```python
from build123d import *

# Parameters (mm, degrees)
F0_W     = 76.2
F0_H     = 25.4
F1_DEPTH = 12.7
F2_W     = 12.7
F2_H     = 12.7
F3_DEPTH = 63.5
F4_R     = 3.175
F5_DEPTH = 50.8


with BuildPart() as f1:
    # F0 (on Top) → F1 (new body)
    with BuildSketch(Plane.XY):
        Rectangle(F0_W, F0_H)
    extrude(amount=F1_DEPTH)

    # F2 (on face) → F3 (join)
    with BuildSketch(Plane.XY.offset(12.7)):
        Rectangle(F2_W, F2_H)
    extrude(amount=F3_DEPTH)

    # F4 (on face) → F5 (join)
    with BuildSketch(Plane.XZ.offset(6.35)):
        with Locations((0, 63.5)):
            Circle(F4_R)
    extrude(amount=F5_DEPTH)


solid = f1.part
```
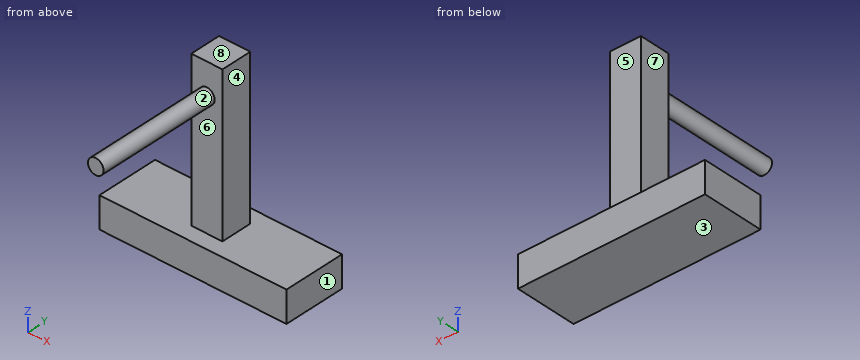
Part model, mm, in its own coordinate system. Face numbers are marked on the shaded views. A direction names the side the tool comes from. Round coordinates to 2 decimals unless told otherwise and drop trailing zeros. Write each loop counter-clockwise with the first axis right and the second up, starting at its lowest first coordinate (ties: lowest second). Pieces come first, ordered by that corner, then holes. Notation, with made-up numbers: (-8.75, 29.25) -> (49.25, 29.25) arc R25 ccw to (49.25, 66.25) -> close; hole circle Ø2 at (87.5, -38.75). An arc over 180 degrees is marked (long way). Return JSON: item names as keys, results as strings. Group by question number.
Q1. Which spindle directions (+Z, -Z, +X, -X, +Y, -Y) get a long thin tool onto all of the face, cutting with end or side? Do the marked faces 1, 2, 3, 4 and 5. Say none if no direction does.
Q2. Saw through at A-A on y = -5. Write the cut outline in (x, z).
Q3. Saw through at C-C on x = 0. Write the cut outline in (y, z) (3 decimals).
Q4. Saw through at B-B on z = 63.5. Write the cut outline in (x, y) (3 decimals), plus the area to 3 significant figures.
Q5. Mould opens along Z. For the marked faces 6, 7 and 8 say: pulls with the +Z half, pulls with the -Z half, needs draft (parallel to the pull), parting line crosses it, or undercut.
Q6. Probe L1, parallel to Z at x = -9.5, y = -2; L2, parallel to X at y = -3.5, z = 31.5. List the from-to ranges inside material, lowest first. Write a range as [from, to].
Q7. Saw through at D-D on y = -39. Write the cut outline in (x, z) (3 decimals).
Q8. Pin check, flat tips, straight feed: pin 1 (6 mm diameter, centred on x = -17.5, z = 14.5, fed in from -Y); pin 2 (12 mm diameter, centred on x = -3, z = 29, fed in from +Y); pin 3 (4 mm diameter, centred on x = 4, y = -19.5, fed in from -Z); pin 4 (20.5 mm diameter, centred on x = 10, y = -5.5, fed in from +Z). Stop position of each tip, or through.
Answer:
{
 "1": {"face 1": "+Z, -Z, +X, +Y, -Y", "face 2": "-Y", "face 3": "-Z, +X, -X, +Y, -Y", "face 4": "+Z, +X, +Y, -Y", "face 5": "+Z, +X, -X, +Y"},
 "2": {"outline": "(-38.1, 0) -> (38.1, 0) -> (38.1, 12.7) -> (6.35, 12.7) -> (6.35, 76.2) -> (-6.35, 76.2) -> (-6.35, 12.7) -> (-38.1, 12.7) -> close"},
 "3": {"outline": "(-57.15, 60.325) -> (-6.35, 60.325) -> (-6.35, 12.7) -> (-12.7, 12.7) -> (-12.7, 0) -> (12.7, 0) -> (12.7, 12.7) -> (6.35, 12.7) -> (6.35, 76.2) -> (-6.35, 76.2) -> (-6.35, 66.675) -> (-57.15, 66.675) -> close"},
 "4": {"outline": "(-6.35, -6.35) -> (-3.175, -6.35) -> (-3.175, -57.15) -> (3.175, -57.15) -> (3.175, -6.35) -> (6.35, -6.35) -> (6.35, 6.35) -> (-6.35, 6.35) -> close", "area": "484 mm2"},
 "5": {"face 6": "undercut", "face 7": "needs draft", "face 8": "pulls with the +Z half"},
 "6": {"L1": "[0, 12.7]", "L2": "[-6.35, 6.35]"},
 "7": {"outline": "circle Ø6.35 at (0, 63.5)"},
 "8": {"pin 1": "y = -12.7", "pin 2": "y = 6.35", "pin 3": "z = 61.03", "pin 4": "z = 76.2"}
}
